Geometry check sheet. Reference: the model listing, model coordinates, mm. Give positions to 0.01 mm unless a question says otherwise; leave off trailing zeros. Loops run counter-clockwise (first coordinate to the right, second up) from the corner with the lowest first, then second, coordinate; pieces in that order, holes last. Notation, with made-up numbers: (50.5, 82.25) -> (92.5, 82.25) arc R19 ccw to (92.5, 112.25) -> close; hole circle Ø1 at (51.25, -21.5). An arc over 180 degrees is marked (long way). Write item = value, one per line.
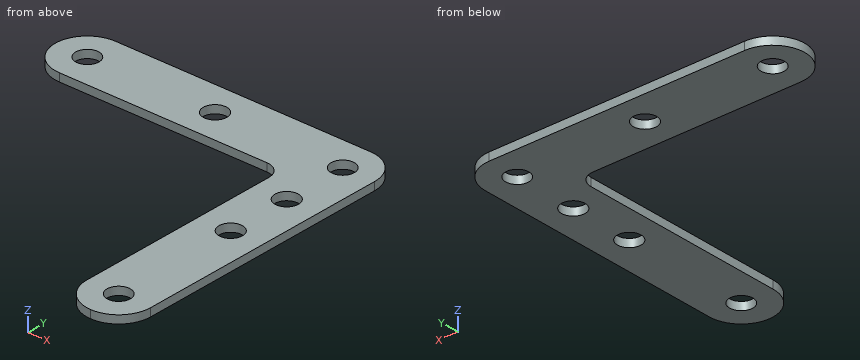
Autodesk Inventor part; units mm, degrees
ref_plane "YZ Plane" through (0, 0, 0) normal (1, 0, 0) x (0, 1, 0)
ref_plane "XZ Plane" through (0, 0, 0) normal (0, 1, 0) x (-1, 0, 0)
ref_plane "XY Plane" through (0, 0, 0) normal (0, 0, 1) x (1, 0, 0)
sketch "Sketch1" plane through (0, 0, 0) normal (0, 0, 1) x (1, 0, 0)
  line L0 (-127.5242, -32.3587) -> (-188.9758, -32.3587)
  line L1 (-128.9881, -97.1287) -> (-187.5119, -97.1287)
  line L2 (-113.8, -97.1287) -> (-113.8, -85.5717)
  circle A0 centre (-120.15, -39.9787) radius 2.3114
  circle A1 centre (-120.15, -90.7787) radius 2.3114
  circle A2 centre (-170.95, -90.7787) radius 2.3114
  circle A3 centre (-170.95, -39.9787) radius 2.3114
  circle A4 centre (-158.25, -39.9787) radius 2.3114
  circle A5 centre (-158.25, -90.7787) radius 2.3114
  circle A6 centre (-120.15, -39.9787) radius 6.35
  circle A7 centre (-170.95, -39.9787) radius 6.35
  circle A8 centre (-170.95, -90.7787) radius 6.35
  circle A9 centre (-120.15, -90.7787) radius 6.35
  line L3 (-170.95, -33.6287) -> (-120.15, -33.6287)
  line L4 (-113.8, -39.9787) -> (-113.8, -90.7787)
  line L5 (-120.15, -97.1287) -> (-170.95, -97.1287)
  line L6 (-170.95, -46.3287) -> (-129.675, -46.3287)
  line L7 (-126.5, -49.5037) -> (-126.5, -81.2537)
  line L8 (-129.675, -84.4287) -> (-170.95, -84.4287)
  arc A10 (-126.5, -49.5037) -> (-129.675, -46.3287) centre (-129.675, -49.5037) ccw
  arc A11 (-129.675, -84.4287) -> (-126.5, -81.2537) centre (-129.675, -81.2537) ccw
  circle A12 centre (-170.95, -39.9787) radius 2.3114
  circle A13 centre (-120.15, -39.9787) radius 2.3114
  circle A14 centre (-120.15, -90.7787) radius 2.3114
  circle A15 centre (-170.95, -90.7787) radius 2.3114
  circle A16 centre (-158.25, -90.7787) radius 2.3114
  circle A17 centre (-158.25, -39.9787) radius 2.3114
  point P0 (0, 0)
  dimension "d6" = 12.7
  dimension "d7" = 12.7
  dimension "d8" = 12.7
  dimension "d9" = 12.7
  dimension "d10" = 3.175
extrude "Extrusion1" add sketch "Sketch1" along normal blind 1.5875
sketch "Sketch2" plane through (0, 0, 1.5875) normal (0, 0, 1) x (1, 0, 0)
  circle A0 centre (-158.25, -39.9787) radius 2.3114
  circle A1 centre (-158.25, -39.9787) radius 2.3114
  circle A2 centre (-158.25, -90.7787) radius 2.3114
  circle A3 centre (-158.25, -90.7787) radius 2.3114
  circle A4 centre (-145.55, -90.7787) radius 2.3368
  circle A5 centre (-170.95, -90.7787) radius 2.3114
  circle A6 centre (-145.55, -39.9787) radius 2.3368
  circle A7 centre (-120.15, -65.3787) radius 2.3368
  circle A8 centre (-120.15, -39.9787) radius 2.3114
  line L0 (-113.8, -90.7787) -> (-113.8, -39.9787)
  circle A9 centre (-170.95, -39.9787) radius 2.3114
  circle A10 centre (-120.15, -90.7787) radius 2.3114
  point P0 (0, 0)
  dimension "d13" = 4.6736
  dimension "d14" = 25.4
  dimension "d15" = 4.6736
  dimension "d16" = 4.6736
  dimension "d17" = 25.4
  dimension "d18" = 6.35
  dimension "d23" = 25.4
  dimension "d24" = 25.4
  dimension "d25" = 25.4
extrude "Extrusion2" cut sketch "Sketch2" against normal blind 25.4 contours A4 | A6 | A7
extrude "Extrusion3" add sketch "Sketch2" against normal up to surface (1.5875 mm away) contours A0 | A2
sketch "Sketch3" plane through (0, 0, 1.5875) normal (0, 0, 1) x (1, 0, 0)
  line L0 (-126.5, -49.5037) -> (-126.5, -81.2537)
  line L1 (-126.5, -81.2537) -> (-126.5, -90.7787)
  line L2 (-170.95, -97.1287) -> (-120.15, -97.1287)
  circle A0 centre (-145.55, -90.7787) radius 2.3368
  circle A1 centre (-145.55, -39.9787) radius 2.3368
  circle A2 centre (-120.15, -65.3787) radius 2.3368
  line L3 (-113.8, -90.7787) -> (-113.8, -39.9787)
  arc A3 (-113.8, -39.9787) -> (-120.15, -33.6287) centre (-120.15, -39.9787) ccw
  line L4 (-120.15, -33.6287) -> (-170.95, -33.6287)
  arc A4 (-170.95, -33.6287) -> (-170.95, -46.3287) centre (-170.95, -39.9787) ccw
  line L5 (-170.95, -46.3287) -> (-129.675, -46.3287)
  arc A5 (-126.5, -49.5037) -> (-129.675, -46.3287) centre (-129.675, -49.5037) ccw
  line L6 (-126.5, -49.5037) -> (-126.5, -81.2537)
  arc A6 (-129.675, -84.4287) -> (-126.5, -81.2537) centre (-129.675, -81.2537) ccw
  line L7 (-129.675, -84.4287) -> (-170.95, -84.4287)
  arc A7 (-170.95, -84.4287) -> (-170.95, -97.1287) centre (-170.95, -90.7787) ccw
  line L8 (-170.95, -97.1287) -> (-120.15, -97.1287)
  arc A8 (-120.15, -97.1287) -> (-113.8, -90.7787) centre (-120.15, -90.7787) ccw
  circle A9 centre (-170.95, -39.9787) radius 2.3114
  circle A10 centre (-120.15, -39.9787) radius 2.3114
  circle A11 centre (-170.95, -90.7787) radius 2.3114
  circle A12 centre (-120.15, -90.7787) radius 2.3114
  arc A13 (-120.15, -97.1287) -> (-113.8, -90.7787) centre (-120.15, -90.7787) ccw
  line L9 (-120.15, -97.1287) -> (-120.15, -97.1287)
  arc A14 (-126.5, -90.7787) -> (-120.15, -97.1287) centre (-120.15, -90.7787) ccw
  circle A15 centre (-120.15, -52.6787) radius 2.3368
  line L10 (-126.5, -79.1192) -> (-182.8014, -79.1192)
  line L11 (-182.8014, -79.1192) -> (-182.8014, -103.4813)
  line L12 (-182.8014, -103.4813) -> (-126.5, -103.4813)
  line L13 (-126.5, -103.4813) -> (-126.5, -79.1192)
  line L14 (-126.5, -97.1287) -> (-120.15, -97.1287)
  point P0 (0, 0)
  dimension "d26" = 6.35
  dimension "d27" = 4.6736
  dimension "d28" = 38.1
  dimension "d29" = 6.35
extrude "Cut1" cut sketch "Sketch3" against normal blind 1.5875 contours L0 A6 L7 A7 L2 L13 L12 L11 L10 | L1 L13 L2 A7 L7 A6
sketch "Sketch4" plane through (0, 0, 1.5875) normal (0, 0, 1) x (1, 0, 0)
  circle A0 centre (-120.15, -52.6787) radius 2.3368
  line L0 (-113.8, -90.7787) -> (-113.8, -39.9787)
  circle A1 centre (-120.15, -90.7787) radius 2.3114
  point P0 (0, 0)
  dimension "d33" = 4.6736
  dimension "d34" = 6.35
  dimension "d35" = 38.1
extrude "Cut2" cut sketch "Sketch4" against normal blind 1.5875 contours A0
fillet "Corner Round1" radius 6.35 1 edges at (-126.5, -97.1287, 0.7937)
equation "\"d31\" = Thickness"
equation "\"d36\" = Thickness"
equation "\"BendRadius\" = Thickness"
equation "\"BendReliefWidth\" = Thickness"
equation "\"BendReliefDepth\" = 0.5 * Thickness"
equation "\"CornerReliefSize\" = 4 * Thickness"
equation "\"MinimumRemnant\" = 2 * Thickness"
equation "\"TransitionRadius\" = BendRadius"
equation "\"JacobiRadiusSize\" = BendRadius"
equation "\"GapSize\" = Thickness"
equation "\"d30\" = Thickness"
properties part number "frontgusset" material "Polycarbonate, Clear"
Item 1: Section check D-D, the plane y = -72.5. Record the cut outline in (x, z).
Answer:
outline = (-126.5, 0) -> (-113.8, 0) -> (-113.8, 1.59) -> (-126.5, 1.59) -> close
Item 2: Thickness scan on L1, parallel to Y at x = -120.15, z = 0.65; L2, parallel to Y at x = -145.55, z = 0.75; L3, parallel to Y at x = -170.95, z = 0.4. Record the ranges inside material, lowest first. Write a range as [from, to].
Answer:
L1 = [-97.13, -93.09], [-88.47, -67.72], [-63.04, -55.02], [-50.34, -42.29], [-37.67, -33.63]
L2 = [-46.33, -42.32], [-37.64, -33.63]
L3 = [-46.33, -42.29], [-37.67, -33.63]
Item 3: Section check A-A, the plane x = -145.55. Record the cut outline in (y, z).
Answer:
outline = (-46.33, 0) -> (-42.32, 0) -> (-42.32, 1.59) -> (-46.33, 1.59) -> close; (-37.64, 0) -> (-33.63, 0) -> (-33.63, 1.59) -> (-37.64, 1.59) -> close
Item 4: Section check B-B, the plane z = 0.3. Give the number of separate pieces and of enclosed holes in the cut face, plus the area to 3 significant figures.
Answer:
separate_pieces = 1
enclosed_holes = 6
area = 1,310 mm^2
Item 5: Section check C-C, the plane x = -155.5. Record the cut outline in (y, z), plus the area to 3 significant figures.
Answer:
outline = (-46.33, 0) -> (-33.63, 0) -> (-33.63, 1.59) -> (-46.33, 1.59) -> close
area = 20.2 mm^2
